Design review of the part built by this model. Coordinates are the model's own, in mm. Round coordinates to 2 decimals unless told otherwise and drop trailing zeros. Write each loop counter-clockwise with the first axis right and the second up, starting at its lowest first coordinate (ties: lowest second). Pieces come first, ordered by that corner, then holes. Notation, with made-up numbers: (-35.75, 59) - (-2.75, 59) arc R21 cw to (-2.75, 95) - close; hole circle Ø10 at (21.25, 26.5). An arc over 180 degrees is marked (long way). Use one line per item in the form item = value.
```python
from build123d import *
from build123d.topology import SkipClean

# Parameters (mm, degrees)
SKETCH_2_R      = 1.6
EXTRUDE_1_DEPTH = 3
EXTRUDE_START   = 3
SKETCH_3_R      = 1.6
EXTRUDE_2_DEPTH = 3
EXTRUDE_START_2 = 5
SKETCH_4_R      = 1.6
EXTRUDE_3_DEPTH = 5


with BuildPart() as part:
    # 草图2 → 凸台-拉伸1 (new body)
    with BuildSketch(Plane(origin=(0, 0, 0), x_dir=(1, 0, 0), z_dir=(0, 1, 0))):
        with BuildLine():
            Line((0, 0), (26, 0))
            Line((26, 0), (26, 25))
            Line((26, 25), (15.428093073, 34.657887136))
            ThreePointArc((15.428093073, 34.657887136), (13, 35.6), (10.571906927, 34.657887136))
            Line((10.571906927, 34.657887136), (0, 25))
            Line((0, 25), (0, 0))
        make_face()
        with Locations(Location((8, 22, 0), (0, 0, 270))):
            Circle(SKETCH_2_R, mode=Mode.SUBTRACT)
        with Locations(Location((18, 22, 0), (0, 0, 90))):
            Circle(SKETCH_2_R, mode=Mode.SUBTRACT)
        with Locations(Location((18, 3, 0), (0, 0, 270))):
            Circle(SKETCH_2_R, mode=Mode.SUBTRACT)
        with Locations(Location((8, 3, 0), (0, 0, 90))):
            Circle(SKETCH_2_R, mode=Mode.SUBTRACT)
        with Locations(Location((13, 32, 0), (0, 0, 270))):
            Circle(SKETCH_2_R, mode=Mode.SUBTRACT)
    extrude(amount=EXTRUDE_1_DEPTH)

    # 草图3 → 凸台-拉伸2 (add)
    with SkipClean():  # the faces are left unmerged after this step: merging them gives an invalid solid
        with BuildSketch(Plane.XZ.offset(EXTRUDE_START)):
            with BuildLine():
                Line((2.02996484, -25.5), (23.97003516, -25.5))
                Line((23.97003516, -25.5), (24.644505458, -26.238301982))
                Line((24.644505458, -26.238301982), (15.428093073, -34.657887136))
                ThreePointArc((15.428093073, -34.657887136), (13, -35.6), (10.571906927, -34.657887136))
                Line((10.571906927, -34.657887136), (1.355494542, -26.238301982))
                Line((1.355494542, -26.238301982), (2.02996484, -25.5))
            make_face()
            with Locations(Location((13, -32, 0), (0, 0, 270))):
                Circle(SKETCH_3_R, mode=Mode.SUBTRACT)
        extrude(amount=-EXTRUDE_2_DEPTH)

    # 草图4 → 凸台-拉伸3 (add)
    with SkipClean():  # the faces are left unmerged after this step: merging them gives an invalid solid
        with BuildSketch(Plane.XZ.offset(3).offset(EXTRUDE_START_2)):
            with BuildLine():
                Line((9.6737238, -33.837358605), (10.571906927, -34.657887136))
                ThreePointArc((10.571906927, -34.657887136), (13, -35.6), (15.428093073, -34.657887136))
                Line((15.428093073, -34.657887136), (16.3262762, -33.837358605))
                ThreePointArc((16.3262762, -33.837358605), (14.7315968, -28.61746064), (9.564559196, -30.37588594))
                ThreePointArc((9.564559196, -30.37588594), (9.201888303, -32.119781203), (9.6737238, -33.837358605))
            make_face()
            with Locations(Location((13, -32, 0), (0, 0, 270))):
                Circle(SKETCH_4_R, mode=Mode.SUBTRACT)
        extrude(amount=-EXTRUDE_3_DEPTH)


solid = part.part
```
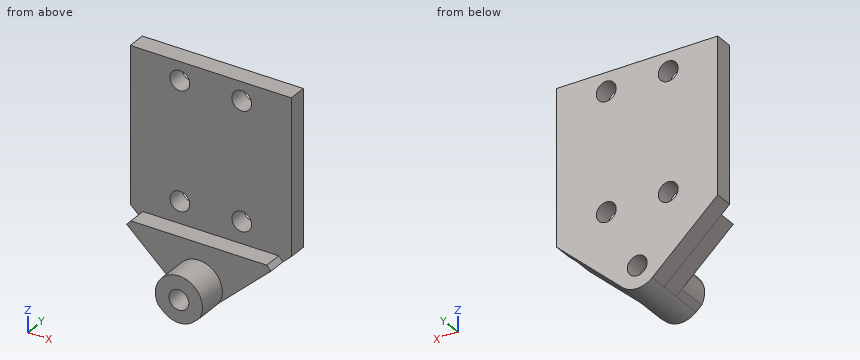
Q1. To check wall thickness, follow line 1 along X through (y, z) = (2.3, -3); line 2 along Z through (x, y) = (18.75, 2.25); line 3 along Y through (x, z) = (13, -3.5). State the ranges of each line that lie inside material, in increasing order. Write a range as from..to.
Calculated:
line_1 = 0..6.4, 9.6..16.4, 19.6..26
line_2 = -31.62..-23.41, -20.59..-4.41, -1.59..0
line_3 = 0..3
Q2. For P1, Ø6, axis at y = -5, z = -20.5, coming from the +X side; P2, Ø3.5, axis at x = 8, z = -22, coming from the -Y side; P3, Ø1.5, axis at x = 18, y = -1.5, coming from the +Z side; P4, Ø5, axis at x = 10.5, z = -24, coming from the -Y side, all flat-tipped, find the tip position at first contact; note any pin that passes through.
Calculated:
P1 = through
P2 = 0
P3 = -25.5
P4 = -3
Q3. We need section D-D on z = -22. Write out the cut boundary in (x, y).
Calculated:
outline = (0, 0) - (6.4, 0) - (6.4, 3) - (0, 3) - close; (9.6, 0) - (16.4, 0) - (16.4, 3) - (9.6, 3) - close; (19.6, 0) - (26, 0) - (26, 3) - (19.6, 3) - close
Q4. We need section B-B on x = 13. Write out the cut boundary in (y, z).
Calculated:
outline = (-8, -35.6) - (3, -35.6) - (3, -33.6) - (-8, -33.6) - close; (-8, -30.4) - (3, -30.4) - (3, 0) - (0, 0) - (0, -25.5) - (-3, -25.5) - (-3, -28.2) - (-8, -28.2) - close
Q5. We need section C-C on y = 1.5. Write out the cut boundary in (x, z), then the cut area to 3 significant figures.
Calculated:
outline = (0, -25) - (10.57, -34.66) arc R3.6 ccw to (15.43, -34.66) - (26, -25) - (26, 0) - (0, 0) - close; hole circle Ø3.2 at (8, -22); hole circle Ø3.2 at (8, -3); hole circle Ø3.2 at (13, -32); hole circle Ø3.2 at (18, -22); hole circle Ø3.2 at (18, -3)
area = 762 mm2
Q6. We need section A-A on y = -2. Write out the cut boundary in (x, z).
Calculated:
outline = (1.36, -26.24) - (10.57, -34.66) arc R3.6 ccw to (15.43, -34.66) - (24.64, -26.24) - (23.97, -25.5) - (2.03, -25.5) - close; hole circle Ø3.2 at (13, -32)
